Study the drawing (mm; zero at the part's minimum x, y, z) and answer. Round coordinates to 2 decimals unless told otherwise and drop trailing zeros. Order: outer loops, then holes, each group sorted by start corner. A loop starts at its lowest first (then second) coordinate and runs counter-clockwise, first axis right, second up. Notation, with made-up numbers: (68, -0.75) - (109, -0.75) arc R3 cw to (109, 4.25) - close; hole circle Ø10 at (17.25, 85.5). An arc over 180 degrees is marked (long way). Put each result on its own line as item: value. Start each with the question number.
Q1. Section C-C on z = 78.5 is taken. Give the vertices of the cut face in (x, y), then the cut area to 3 significant figures.
Q2. This flat-tipped pin is pushed along its axis until it touches: pin 1 Ø2 at (x, z) = (33, 39) entering from -Y. Where does it stop, or does it pass through?
Q3. Section D-D on x = 78.5 is taken. Give the vertices of the cut face in (y, z).
Q4. Section B-B on x = 40.5 is taken. Give the vertices of the cut face in (y, z).
Q5. Find the intervals of material crossed by line 1 along X through (y, z) = (1.05, 40.5); line 2 along X through (y, z) = (0.7, 58); line 3 along Z through (x, y) = (66, 1.35), in increasing order. Write a range as from..to.
Q6. Section A-A on z = 40.5 is taken. Give the vertices of the cut face in (x, y), then the cut area to 3 significant figures.
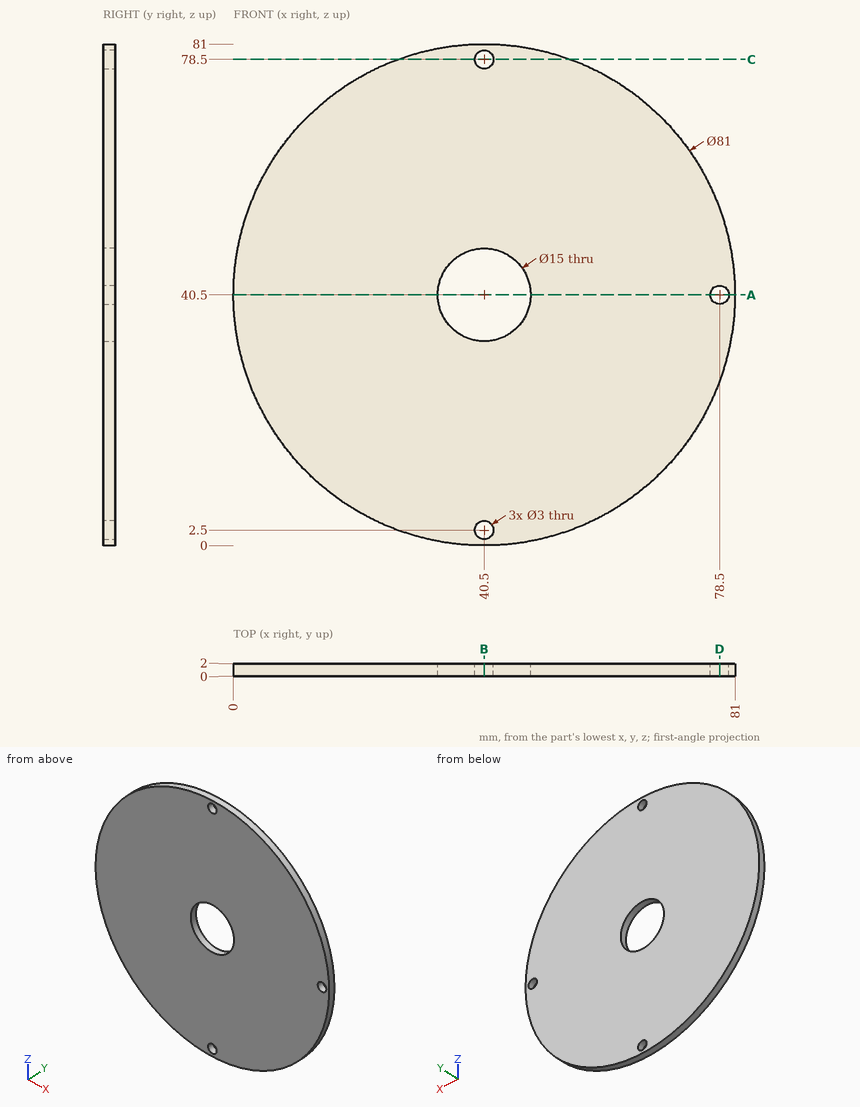
Findings:
1. outline: (26.49, 0) - (39, 0) - (39, 2) - (26.49, 2) - close; (42, 0) - (54.51, 0) - (54.51, 2) - (42, 2) - close
1. area: 50.0 mm2
2. pin 1: y = 0
3. outline: (0, 26.49) - (2, 26.49) - (2, 39) - (0, 39) - close; (0, 42) - (2, 42) - (2, 54.51) - (0, 54.51) - close
4. outline: (0, 0) - (2, 0) - (2, 1) - (0, 1) - close; (0, 4) - (2, 4) - (2, 33) - (0, 33) - close; (0, 48) - (2, 48) - (2, 77) - (0, 77) - close; (0, 80) - (2, 80) - (2, 81) - (0, 81) - close
5. line 1: 0..33, 48..77, 80..81
5. line 2: 3.98..77.02
5. line 3: 9.04..71.96
6. outline: (0, 0) - (33, 0) - (33, 2) - (0, 2) - close; (48, 0) - (77, 0) - (77, 2) - (48, 2) - close; (80, 0) - (81, 0) - (81, 2) - (80, 2) - close
6. area: 126 mm2
